The listing builds one solid part. Answer for the finished solid, in the listing's coordinates (mm). Round coordinates to 2 decimals unless told otherwise and drop trailing zeros. Answer in a Markdown table with one row per item. Add a question column.
```python
from build123d import *

# Parameters (mm, degrees)
F2_DEPTH = 6.35
F3_R     = 3.175
F4_DEPTH = 6.351


with BuildPart() as f2:
    # F1 (on Front) → F2 (new body)
    with BuildSketch(Plane.XZ):
        with BuildLine():
            add(Edge.make_bspline(
                [(6.055434, -26.960964), (36.11994, -9.76876), (142.355109, 21.639892), (157.20883, 71.411878)],
                knots=[6.343497, 6.343497, 6.343497, 6.343497, 183.773328, 183.773328, 183.773328, 183.773328], degree=3))
            add(Edge.make_bspline(
                [(157.20883, 71.411878), (140.229825, 76.100313), (59.48711, 41.521585), (-10.778349, 4.286915)],
                knots=[0, 0, 0, 0, 180.643576, 180.643576, 180.643576, 180.643576], degree=3))
            add(Edge.make_bspline(
                [(-10.778349, 4.286915), (-16.87327, 1.05713), (-22.889359, -2.192639), (-28.778164, -5.438497)],
                knots=[180.643576, 180.643576, 180.643576, 180.643576, 196.312844, 196.312844, 196.312844, 196.312844], degree=3))
            add(Edge.make_bspline(
                [(-28.778164, -5.438497), (-70.206457, -28.273415), (-105.335108, -50.91478), (-117.293463, -65.042991)],
                knots=[196.312844, 196.312844, 196.312844, 196.312844, 306.547615, 306.547615, 306.547615, 306.547615], degree=3))
            Line((-117.293463, -65.042991), (-114.262126, -80.902003))
            Line((-114.262126, -80.902003), (-90.068042, -88.572152))
            add(Edge.make_bspline(
                [(-90.068042, -88.572152), (-73.63602, -64.229396), (-41.701322, -45.705485), (-27.396359, -42.834848)],
                knots=[0, 0, 0, 0, 77.586345, 77.586345, 77.586345, 77.586345], degree=3))
            ThreePointArc((-27.396359, -42.834848), (-16.306206, -33.145092), (-2.016447, -36.706783))
            Line((-2.016447, -36.706783), (-2.007486, -36.692901))
            ThreePointArc((-2.007486, -36.692901), (1.519559, -36.7814), (2.950716, -33.556547))
            ThreePointArc((2.950716, -33.556547), (3.46235, -29.768859), (6.055434, -26.960964))
        make_face()
        with BuildLine():
            add(Edge.make_bspline(
                [(-10.778349, 4.286915), (-16.87327, 1.05713), (-22.889359, -2.192639), (-28.778164, -5.438497)],
                knots=[180.643576, 180.643576, 180.643576, 180.643576, 196.312844, 196.312844, 196.312844, 196.312844], degree=3))
            ThreePointArc((-10.778349, 4.286915), (-14.175572, 3.561969), (-17.44593, 4.733046))
            ThreePointArc((-17.44593, 4.733046), (-20.505455, 5.133112), (-22.537804, 2.811411))
            ThreePointArc((-22.537804, 2.811411), (-24.779979, -1.97768), (-28.778164, -5.438497))
        make_face()
    extrude(amount=F2_DEPTH)

    # F3 (on Front) + F2_face (on face) → F4 (cut, through all)
    with BuildSketch(Plane.XZ):
        with Locations((-101.384849, -69.758254)):
            Circle(F3_R)
        with Locations((-63.452638, -42.958295)):
            Circle(F3_R)
        with Locations((-23.929693, -18.416649)):
            Circle(F3_R)
    with BuildSketch(Plane(origin=(16.779727, -6.35, -3.819099), x_dir=(1, 0, 0), z_dir=(0, -1, 0))):
        with BuildLine():
            ThreePointArc((-13.829011, -29.737449), (-13.317377, -25.94976), (-10.724293, -23.141866))
            add(Edge.make_bspline(
                [(-10.724293, -23.141866), (19.340213, -5.949661), (125.575382, 25.458991), (140.429103, 75.230977)],
                knots=[6.343497, 6.343497, 6.343497, 6.343497, 183.773328, 183.773328, 183.773328, 183.773328], degree=3))
            add(Edge.make_bspline(
                [(140.429103, 75.230977), (123.450098, 79.919412), (42.707383, 45.340683), (-27.558076, 8.106014)],
                knots=[0, 0, 0, 0, 180.643576, 180.643576, 180.643576, 180.643576], degree=3))
            ThreePointArc((-27.558076, 8.106014), (-30.955298, 7.381068), (-34.225657, 8.552144))
            ThreePointArc((-34.225657, 8.552144), (-37.285181, 8.952211), (-39.317531, 6.630509))
            ThreePointArc((-39.317531, 6.630509), (-41.559706, 1.841419), (-45.55789, -1.619399))
            add(Edge.make_bspline(
                [(-45.55789, -1.619399), (-86.986184, -24.454316), (-122.114835, -47.095681), (-134.07319, -61.223893)],
                knots=[196.312844, 196.312844, 196.312844, 196.312844, 306.547615, 306.547615, 306.547615, 306.547615], degree=3))
            Line((-134.07319, -61.223893), (-131.041853, -77.082904))
            Line((-131.041853, -77.082904), (-106.847769, -84.753053))
            add(Edge.make_bspline(
                [(-106.847769, -84.753053), (-90.415747, -60.410298), (-58.481049, -41.886386), (-44.176085, -39.015749)],
                knots=[0, 0, 0, 0, 77.586345, 77.586345, 77.586345, 77.586345], degree=3))
            ThreePointArc((-44.176085, -39.015749), (-33.085933, -29.325993), (-18.796174, -32.887684))
            Line((-18.796174, -32.887684), (-18.787213, -32.873803))
            ThreePointArc((-18.787213, -32.873803), (-15.260168, -32.962301), (-13.829011, -29.737449))
        make_face()
    extrude(amount=F4_DEPTH, mode=Mode.SUBTRACT)


solid = f2.part
```
1. Straight lines are drawn through the part: line 1 along Z through (x, y) = (-25.5, -3); line 2 along Z through (x, y) = (-24, -1.75); line 3 along X through (y, z) = (-1.25, -17.5). For each, find the intervals that lie inside material, in ascending order.
2. The mould has two halves that part along Z. Classify faces 1 (the cylindrical face through (-24.735, -3.131, -1.918)), 2 (the flat face through (-102.334, -3.131, -84.683)), 3 (the cylindrical face through (-61.75, -3.13, -40.28)), 4 (the cylindrical face through (-27.1, -3.13, -18.28)): released by +Z, released by -Z, zero draft, split by the parting line, or undercut.
3. Each of these flat-tipped pins is pushed along its axis until it touches: pin 1 (2 mm diameter, centred on x = -61.5, y = -2.5, fed in from -Z); pin 2 (2 mm diameter, centred on x = -40.5, y = -4, fed in from +Z). Where does it stop, or does it pass through?
4. The part is cut by section A-A (y = -1.5). Give the number of separate pieces and of enclosed holes in the cut face, then the cut area to 3 significant figures.
Report:
| question | item | result |
|---|---|---|
| 1 | line 1 | z = -39.34 to -21.18, -15.66 to -2.85 |
| 1 | line 2 | z = -37.54 to -21.59, -15.24 to -0.82 |
| 1 | line 3 | x = -50.09 to -26.97, -20.89 to 25.88 |
| 2 | face 1 | released by +Z |
| 2 | face 2 | released by -Z |
| 2 | face 3 | undercut |
| 2 | face 4 | undercut |
| 3 | pin 1 | stops at z = -60.88 |
| 3 | pin 2 | stops at z = -11.42 |
| 4 | separate pieces | 1 |
| 4 | enclosed holes | 3 |
| 4 | area | 9,920 mm^2 |
